Part model, mm, in its own coordinate system. Face numbers are marked on the shaded views. A direction names the side the tool comes from. Coordinates: 2 decimals unless noted, no trailing zeros. Write each loop counter-clockwise with the first axis right and the second up, starting at its lowest first coordinate (ties: lowest second). Pieces come first, ordered by that corner, then holes. Notation, with made-up numbers: (-40, 28) - (12, 28) arc R11 cw to (12, 37) - close; hole circle Ø9 at (40.25, 42). An arc over 180 degrees is marked (long way). Write each question's results on one line, items separated by ' | '.
from build123d import *

# Parameters (mm, degrees)
BASE_EXTRUDE_THIN_DEPTH = 88.9
BOSS_EXTRUDE1_REACH     = 193.345
SKETCH2_R               = 34.925
BOSS_EXTRUDE1_DRAFT     = 5
SKETCH3_R               = 26.9875
CUT_EXTRUDE1_DEPTH      = 192.344793501
SKETCH4_R               = 7.9375
CUT_EXTRUDE2_DEPTH      = 190.225738207
RIB1_REACH              = 192.398
SKETCH5_WALLS_W         = 403.925170957
SKETCH5_WALLS_H         = 7.9375
RIB1_DRAFT_ANGLE        = 1


with BuildPart() as part:
    # Sketch1 → Base-Extrude-Thin (new body)
    with BuildSketch(Plane.XY):
        Polygon((0, 38.1), (0, 0), (165.1, 0), (165.1, 12.7), (12.7, 12.7), (12.7, 38.1), align=None)
    extrude(amount=-BASE_EXTRUDE_THIN_DEPTH)




with BuildPart() as boss_extrude1_long_prism_1:
    # Sketch2 → Boss-Extrude1 (the long prism of profile 1, to be tilted and cut off)
    with BuildSketch(Plane(origin=(0, 38.1, 0), x_dir=(-1, 0, 0), z_dir=(0, 1, 0))):
        with Locations((-82.55, -44.45)):
            Circle(SKETCH2_R)
    extrude(amount=-BOSS_EXTRUDE1_REACH)
    boss_extrude1_tool1_sides = [boss_extrude1_long_prism_1.faces().sort_by_distance(p)[0] for p in [
        (117.475, -58.5725, -44.45),
    ]]
    draft(boss_extrude1_tool1_sides, Plane(origin=(0, 38.1, 0), x_dir=(-1, 0, 0), z_dir=(0, 1, 0)), BOSS_EXTRUDE1_DRAFT)  # the draft: side faces tilted about the start plane


with BuildPart() as part_1:
    add(part.part)
    boss_extrude1_tool1 = boss_extrude1_long_prism_1.part - part.part
    add(boss_extrude1_tool1.solids().sort_by_distance((82.55, 38.1, -44.45))[0])

    # Sketch3 → Cut-Extrude1 (cut, through all)
    with BuildSketch(Plane(origin=(0, 38.1, 0), x_dir=(-1, 0, 0), z_dir=(0, 1, 0))):
        with Locations(Location((-82.55, -44.45, 0), (0, 0, 90))):
            Circle(SKETCH3_R)
    extrude(amount=-CUT_EXTRUDE1_DEPTH, mode=Mode.SUBTRACT)

    # Sketch4 → Cut-Extrude2 (cut, through all)
    with BuildSketch(Plane(origin=(0, 12.7, 0), x_dir=(-1, 0, 0), z_dir=(0, 1, 0))):
        with Locations(Location((-149.225, -15.875, 0), (0, 0, 90))):
            Circle(SKETCH4_R)
        with Locations(Location((-149.225, -73.025, 0), (0, 0, 90))):
            Circle(SKETCH4_R)
    extrude(amount=-CUT_EXTRUDE2_DEPTH, mode=Mode.SUBTRACT)

    # Sketch5 walls → Rib1 (add, up to next)
    with BuildSketch(Plane(origin=(0, 33.02, 0), x_dir=(-1, 0, 0), z_dir=(0, 1, 0)), mode=Mode.PRIVATE) as rib1_sk1:
        with Locations((-32.214634147, -44.45)):
            Rectangle(SKETCH5_WALLS_W, SKETCH5_WALLS_H)
    rib1_tool1 = extrude(rib1_sk1.sketch, amount=-RIB1_REACH, mode=Mode.PRIVATE) - part_1.part
    add(rib1_tool1.solids().sort_by_distance((32.214634146, 33.02, -44.45))[0])

    # Rib1 draft
    rib1_draft_faces = [part_1.faces().sort_by_distance(p)[0] for p in [
        (32.214634147, 32.52, -48.41875),
        (32.214634147, 32.52, -40.48125),
    ]]
    draft(rib1_draft_faces, Plane(origin=(32.214634146, 33.02, -44.45), x_dir=(-1, 0, 0), z_dir=(0, 1, 0)), RIB1_DRAFT_ANGLE)


solid = part_1.part
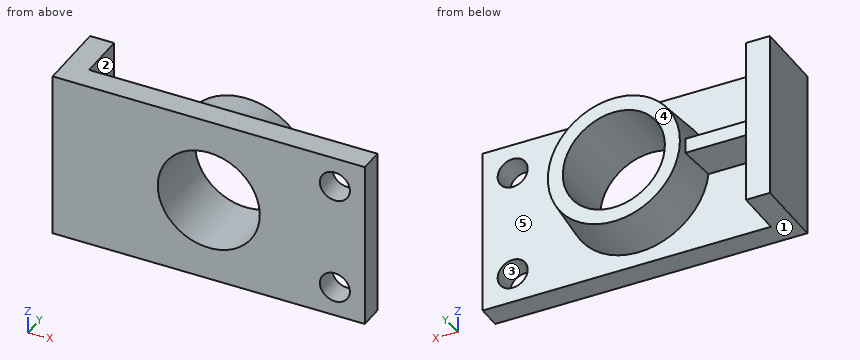
(1) Saw through at A-A on x = 82.55. Write the cut outline in (y, z) (1 decimal).
Return value:
outline: (0, -88.9) - (12.7, -88.9) - (12.7, -81.6) - (38.1, -79.4) - (38.1, -71.4) - (0, -71.4) - close; (0, -17.5) - (38.1, -17.5) - (38.1, -9.5) - (12.7, -7.3) - (12.7, 0) - (0, 0) - close
(2) Two-plate mould, pull along Z, no slides. Class the marked faces 1, 2 and 3: released by +Z, released by -Z, zero draft, split by the parting line, or undercut.
Return value:
face 1: released by -Z | face 2: zero draft | face 3: undercut
(3) 3-axis set-ups, long thin cutter, end or side, ignore diameter. For the marked faces 4 and 5: which of +Z, -Z, +X, -X, +Y, -Y reach the whole face in a straight line?
Return value:
face 4: +Z, -Z, +X, -X, +Y | face 5: +Y
(4) Saw through at C-C on x = 155. Write the cut outline in (y, z), then the cut area to 3 significant figures.
Return value:
outline: (0, -88.9) - (12.7, -88.9) - (12.7, -78.47) - (0, -78.47) - close; (0, -67.58) - (12.7, -67.58) - (12.7, -21.32) - (0, -21.32) - close; (0, -10.43) - (12.7, -10.43) - (12.7, 0) - (0, 0) - close | area: 852 mm^2
(5) Wall check: line 1 (X direction, y = 30, z = -24); line 2 (X direction, y = 9, z = -44.45); line 3 (X direction, y = 20, z = -65.5). Give the ranges that are in metal, low to high. Write a range as from..to.
Return value:
line 1: x = 0..12.7, 53.37..64.94, 100.16..111.73 | line 2: x = 0..55.56, 109.54..165.1 | line 3: x = 0..12.7, 52.72..65.66, 99.44..112.38
(6) Saw through at B-B on y = 35. Count the separate pieces of the cut face and the enclosed holes in it, then the cut area to 3 significant figures.
Return value:
separate pieces: 2 | enclosed holes: 1 | area: 2,730 mm^2
(7) Flat gauge pins, fed straight in: P1, Ø8.5, axis at x = 37, z = -43, coming from the +Y side; P2, Ø12, axis at x = 126.5, z = -53.5, coming from the +Y side; P3, Ø2, axis at x = 108.5, z = -68.5, coming from the -Y side; P4, Ø8, axis at x = 119.5, y = 23, coming from the +Z side. Where does each tip first touch, or does it go through?
Return value:
P1: stops at y = 33.02 | P2: stops at y = 12.7 | P3: stops at y = 0 | P4: stops at z = -29.31
